For this review, use the dimensioned drawing (mm, ordinates from the lowest corner) and the shaded views. A direction names the side the tool comes from. Round coordinates to 2 decimals unless told otherwise and drop trailing zeros. Order: outer loops, then holes, each group sorted by start corner. A loop starts at its lowest first (then second) coordinate and runs counter-clockwise, first axis right, second up. Notation, with made-up numbers: (62, 25) - (72, 25) arc R22 ccw to (72, 56) - close; hole circle Ø10 at (-3.75, 62.5). An arc over 180 degrees is marked (long way). Write each question's results on one line, items separated by ' | '. Start each with the question number.
(1) Take a section at A-A, the plane x = 2.5. Give the boundary of the cut face in (y, z).
(2) Take a section at B-B, the plane y = 2.5. Give the boundary of the cut face in (x, z), plus the area to 3 significant figures.
(3) For L1, parallel to Y at x = 2.35, z = 17.5; L2, parallel to Z at x = 1.35, y = 6.5; L3, parallel to Z at x = 3.55, y = 9.5, list the stretches that pass through material, from the lowest coordinate up. Write a range as from..to.
(4) Insertion check: pin 1 Ø1 at (x, y) = (4, 3) entering from -Z; pin 2 Ø2 at (x, z) = (0.5, 18.5) entering from -Y. Each pin has a flat end and moves straight along its axis. Give the tip position at first contact, or say it passes through.
(5) Take a section at D-D, the plane x = 3.85. Give the boundary of the cut face in (y, z).
(6) For the marked faces 1, 2, 3 and 4, list the 3-axis set-ups (+Z, -Z, +X, -X, +Y, -Y) from which the entire face can be reached by the end or side of a thin tool; tool diameter is ignored.
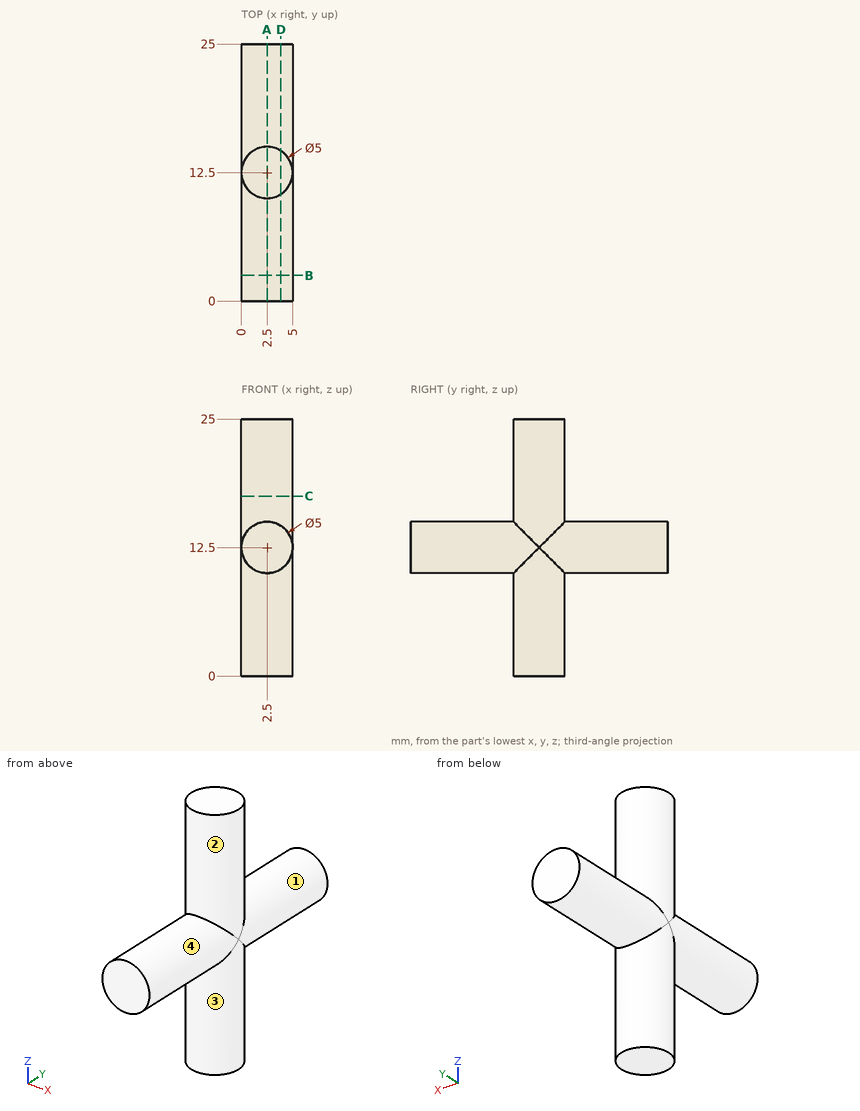
Results below:
1) outline: (0, 10) - (10, 10) - (10, 0) - (15, 0) - (15, 10) - (25, 10) - (25, 15) - (15, 15) - (15, 25) - (10, 25) - (10, 15) - (0, 15) - close
2) outline: circle Ø5 at (2.5, 12.5) | area: 19.6 mm^2
3) L1: y = 10..15 | L2: z = 10.28..14.72 | L3: z = 10.23..14.77
4) pin 1: stops at z = 10.21 | pin 2: stops at y = 10.21
5) outline: (0, 10.4) - (10.4, 10.4) - (10.4, 0) - (14.6, 0) - (14.6, 10.4) - (25, 10.4) - (25, 14.6) - (14.6, 14.6) - (14.6, 25) - (10.4, 25) - (10.4, 14.6) - (0, 14.6) - close
6) face 1: +Y | face 2: +Z | face 3: -Z | face 4: -Y
